Geometry: see drawing. Coordinates: mm, zero at the bounding-box minimum. Round coordinates to 2 decimals unless told otherwise and drop trailing zeros. Loops run counter-clockwise (first coordinate to the right, second up) from the corner with the lowest first, then second, coordinate; pieces in that order, holes last.
(1) Material intervals for probe 1 along X at (y, z) = (4, 4); probe 2 along Y at (x, z) = (50.5, 4.55); probe 3 along Y at (x, z) = (108, 3.9), sorted ascending.
(2) Section D-D, the plane x = 14. Return the cut outline in (y, z).
(3) Section C-C, the plane z = 2.4. Count the separate pieces of the cut face and the enclosed holes in it, plus the area to 4 significant figures.
(4) Section B-B, the plane y = 23.5. Return the cut outline in (x, z).
(5) First-contact query: pin 1 Ø3 at (x, z) = (54.5, 3.5) entering from -Y; pin 2 Ø1.5 at (x, z) = (45.5, 2) entering from -Y; pin 3 Ø1.5 at (y, z) = (38, 3) entering from +X; pin 4 Ø2.5 at (x, z) = (2, 1.5) entering from +Y. Flat tips, straight axial feed; report the tip coordinate or a pass-through.
(6) Section A-A, the plane x = 117. Return the cut outline in (y, z), plus the area to 3 significant figures.
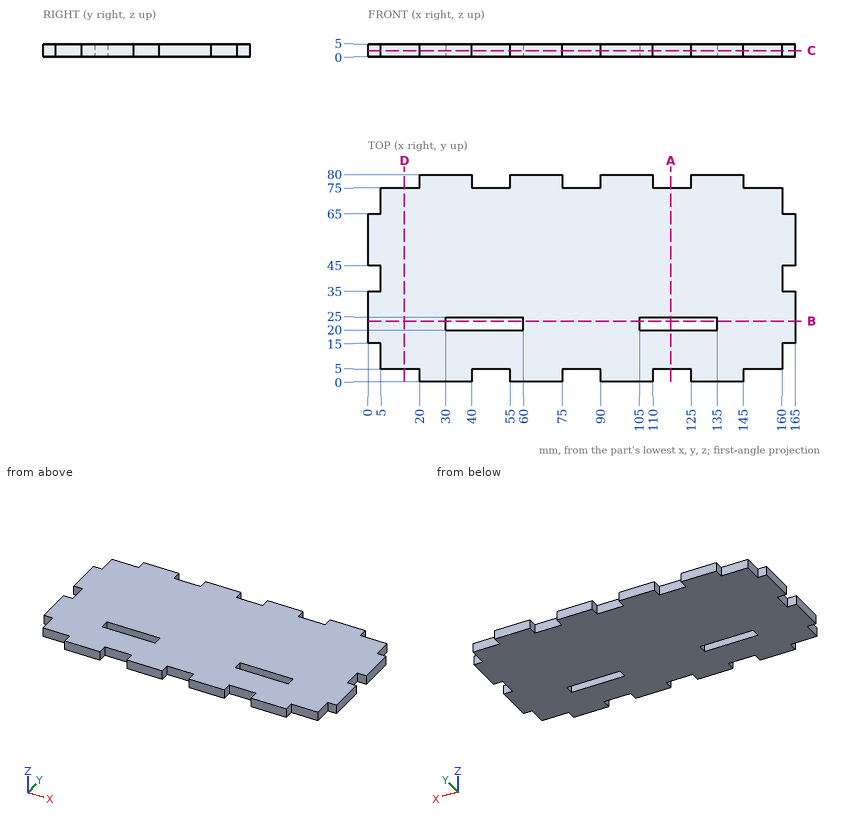
Output values:
1. probe 1: x = 20 to 40, 55 to 75, 90 to 110, 125 to 145
1. probe 2: y = 5 to 20, 25 to 75
1. probe 3: y = 0 to 20, 25 to 80
2. outline: (5, 0) - (75, 0) - (75, 5) - (5, 5) - close
3. separate pieces: 1
3. enclosed holes: 2
3. area: 11,750 mm2
4. outline: (0, 0) - (30, 0) - (30, 5) - (0, 5) - close; (60, 0) - (105, 0) - (105, 5) - (60, 5) - close; (135, 0) - (165, 0) - (165, 5) - (135, 5) - close
5. pin 1: stops at y = 0
5. pin 2: stops at y = 5
5. pin 3: stops at x = 160
5. pin 4: stops at y = 65
6. outline: (5, 0) - (20, 0) - (20, 5) - (5, 5) - close; (25, 0) - (75, 0) - (75, 5) - (25, 5) - close
6. area: 325 mm2
